Geometry check sheet. Reference: the model listing, model coordinates, mm. Give positions to 0.01 mm unless a question says otherwise; leave off trailing zeros. Write each loop counter-clockwise with the first axis right and the second up, starting at its lowest first coordinate (ties: lowest second). Pieces come first, ordered by that corner, then holes. Notation, with made-up numbers: (17.25, -13) -> (27.25, -13) arc R14 cw to (27.25, -9) -> close; hole circle Ø2 at (87, 2). An arc over 180 degrees is marked (long way). One line per item, written item: value.
from build123d import *

# Parameters (mm, degrees)
F0_R     = 3.25
F1_DEPTH = 1
F2_R     = 3.25
F3_DEPTH = 1
F4_R     = 3.25
F5_DEPTH = 1
F6_SIZE  = 0.4


with BuildPart() as f1:
    # F0 (on Top) → F1 (new body)
    with BuildSketch(Plane.XY):
        with BuildLine():
            Line((32.5, 15), (-32.5, 15))
            ThreePointArc((-32.5, 15), (-36.035534, 13.535534), (-37.5, 10))
            Line((-37.5, 10), (-37.5, -10))
            ThreePointArc((-37.5, -10), (-36.035534, -13.535534), (-32.5, -15))
            Line((-32.5, -15), (32.5, -15))
            ThreePointArc((32.5, -15), (36.035534, -13.535534), (37.5, -10))
            Line((37.5, -10), (37.5, 10))
            ThreePointArc((37.5, 10), (36.035534, 13.535534), (32.5, 15))
        make_face()
        with Locations((-27.5, 0)):
            Circle(F0_R, mode=Mode.SUBTRACT)
    extrude(amount=F1_DEPTH)

    # F2 (on face) → F3 (join)
    with BuildSketch(Plane.XY.offset(1)):
        with BuildLine():
            Line((12.5, 15), (-32.5, 15))
            ThreePointArc((-32.5, 15), (-36.035534, 13.535534), (-37.5, 10))
            Line((-37.5, 10), (-37.5, -10))
            ThreePointArc((-37.5, -10), (-36.035534, -13.535534), (-32.5, -15))
            Line((-32.5, -15), (12.5, -15))
            ThreePointArc((12.5, -15), (16.035534, -13.535534), (17.5, -10))
            Line((17.5, -10), (17.5, 10))
            ThreePointArc((17.5, 10), (16.035534, 13.535534), (12.5, 15))
        make_face()
        with Locations((-27.5, 0)):
            Circle(F2_R, mode=Mode.SUBTRACT)
    extrude(amount=F3_DEPTH)

    # F4 (on face) → F5 (join)
    with BuildSketch(Plane.XY.offset(2)):
        with BuildLine():
            Line((-7.5, 15), (-32.5, 15))
            ThreePointArc((-32.5, 15), (-36.035534, 13.535534), (-37.5, 10))
            Line((-37.5, 10), (-37.5, -10))
            ThreePointArc((-37.5, -10), (-36.035534, -13.535534), (-32.5, -15))
            Line((-32.5, -15), (-7.5, -15))
            ThreePointArc((-7.5, -15), (-3.964466, -13.535534), (-2.5, -10))
            Line((-2.5, -10), (-2.5, 10))
            ThreePointArc((-2.5, 10), (-3.964466, 13.535534), (-7.5, 15))
        make_face()
        with Locations((-27.5, 0)):
            Circle(F4_R, mode=Mode.SUBTRACT)
    extrude(amount=F5_DEPTH)

    # F6
    f6_edges = [f1.edges().sort_by_distance(p)[0] for p in [
        (-30.75, 0, 3),
        (-30.75, 0, 0),
    ]]
    chamfer(f6_edges, length=F6_SIZE)


solid = f1.part
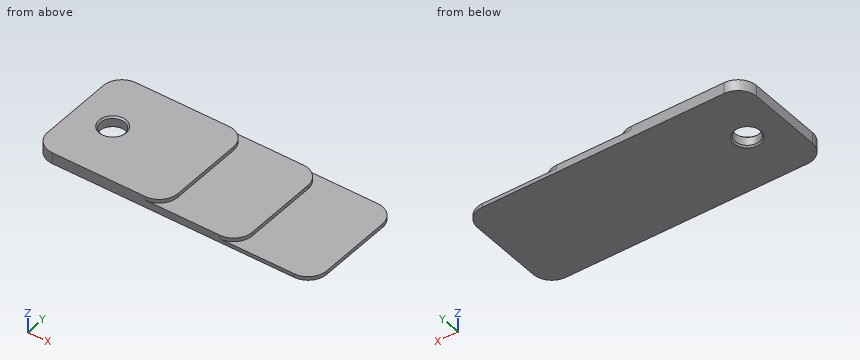
1) Sectioned sample at C-C on y = 5.5. Record the cut outline in (x, z), plus the area to 3 significant figures.
Verdict:
outline: (-37.5, 0) -> (37.5, 0) -> (37.5, 1) -> (17.5, 1) -> (17.5, 2) -> (-2.5, 2) -> (-2.5, 3) -> (-37.5, 3) -> close
area: 165 mm^2
2) Depth check by flat-ended pin: pin 1 Ø1.5 at (y, z) = (11, 1.5) entering from -X; pin 2 Ø1.1 at (y, z) = (-4, 2.5) entering from +X; pin 3 Ø7.5 at (x, y) = (24, -5.5) entering from +Z; pin 4 Ø7.5 at (x, y) = (-27.5, 0) entering from -Z. Enter the tip coordinate at first touch or a pass-through.
Verdict:
pin 1: x = -37.49
pin 2: x = 17.5
pin 3: z = 1
pin 4: z = 0
3) Sectioned sample at B-B on y = 0. Record the cut outline in (x, z), plus the area to 3 significant figures.
Verdict:
outline: (-37.5, 0) -> (-31.15, 0) -> (-30.75, 0.4) -> (-30.75, 2.6) -> (-31.15, 3) -> (-37.5, 3) -> close; (-24.25, 0.4) -> (-23.85, 0) -> (37.5, 0) -> (37.5, 1) -> (17.5, 1) -> (17.5, 2) -> (-2.5, 2) -> (-2.5, 3) -> (-23.85, 3) -> (-24.25, 2.6) -> close
area: 145 mm^2
4) Sectioned sample at D-D on x = 13.5. Record the cut outline in (y, z), plus the area to 3 significant figures.
Verdict:
outline: (-15, 0) -> (15, 0) -> (15, 1) -> (14.9, 1) -> (14.9, 2) -> (-14.9, 2) -> (-14.9, 1) -> (-15, 1) -> close
area: 59.8 mm^2
5) Scan lines: probe 1 along Y at (x, z) = (-27.5, 1.85); probe 2 along Z at (x, y) = (24.5, 0.5); probe 3 along Z at (x, y) = (3.5, 2). Record each from-to range of solid material in increasing order.
Verdict:
probe 1: -15 to -3.25, 3.25 to 15
probe 2: 0 to 1
probe 3: 0 to 2
6) Sectioned sample at A-A on x = -27.5. Record the cut outline in (y, z), plus the area to 3 significant figures.
Verdict:
outline: (-15, 0) -> (-3.65, 0) -> (-3.25, 0.4) -> (-3.25, 2.6) -> (-3.65, 3) -> (-15, 3) -> close; (3.25, 0.4) -> (3.65, 0) -> (15, 0) -> (15, 3) -> (3.65, 3) -> (3.25, 2.6) -> close
area: 70.2 mm^2
